Design review of the part built by this model. Coordinates are the model's own, in mm. Coordinates: 2 decimals unless noted, no trailing zeros. Loops run counter-clockwise (first coordinate to the right, second up) from the corner with the lowest first, then second, coordinate; pieces in that order, holes last. Notation, with made-up numbers: (23.5, 88) - (52.5, 88) arc R19 ccw to (52.5, 104) - close; hole circle Ø10 at (19.25, -9). An arc over 180 degrees is marked (long way). Use one line per item in the form item = value. Start each with the question number.
(1) Add section C-C (z = -7). Count the separate pieces of the cut face and the enclosed holes in it, plus the area to 4 significant figures.
(2) Add section B-B (x = 36.25). State the section outline as (y, z) points, plus the area to 3 significant figures.
(3) For L1, parallel to Z at x = 36.25, y = 0.65; L2, parallel to Z at x = 42, y = 0.65; L3, parallel to Z at x = 24.5, y = 1.85, list the stretches that pass through material, from the lowest coordinate up.
(4) Add section A-A (x = 16.9). State the section outline as (y, z) points, plus the area to 3 significant figures.
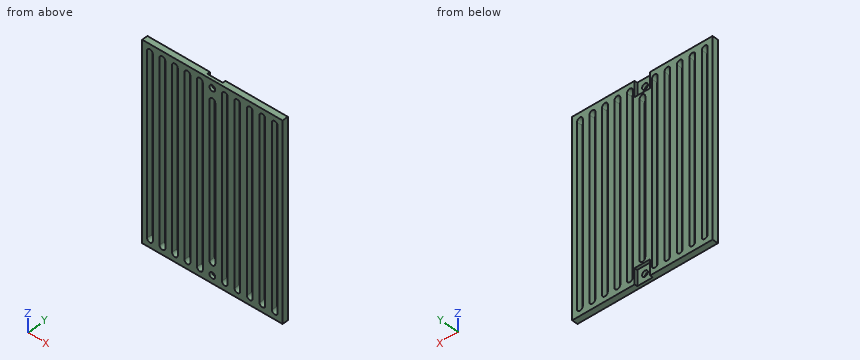
Autodesk Inventor part; units mm, degrees
ref_plane "YZ Plane" through (0, 0, 0) normal (1, 0, 0) x (0, 1, 0)
ref_plane "XZ Plane" through (0, 0, 0) normal (0, 1, 0) x (-1, 0, 0)
ref_plane "XY Plane" through (0, 0, 0) normal (0, 0, 1) x (1, 0, 0)
sketch "Sketch1" plane through (0, 0, 0) normal (0, 1, 0) x (-1, 0, 0)
  line L0 (0, 0) -> (-72.5, 0)
  line L1 (-72.5, 0) -> (-72.5, -100)
  line L2 (-72.5, -100) -> (0, -100)
  line L3 (0, -100) -> (0, 0)
  dimension "d0" = 72.5
  dimension "d1" = 100
extrude "Extrusion1" add sketch "Sketch1" along normal blind 3
sketch "Sketch11" plane through (0, 3, 0) normal (0, 1, 0) x (1, 0, 0)
  point P0 (0, 0)
sketch "Sketch13" plane through (0, 3, 0) normal (0, 1, 0) x (1, 0, 0)
  line L0 (0, 0) -> (72.5, 0)
  line L1 (36.25, 0) -> (36.25, 8)
  line L2 (36.25, 8) -> (32.25, 8)
  line L3 (32.25, 8) -> (32.25, 0)
  line L4 (36.25, 0) -> (32.25, 0)
  line L5 (36.25, 0) -> (40.25, 0)
  line L6 (40.25, 0) -> (40.25, 8)
  line L7 (40.25, 8) -> (36.25, 8)
  line L8 (72.5, 100) -> (0, 100)
  line L9 (36.25, 100) -> (32.25, 100)
  line L10 (32.25, 100) -> (32.25, 92)
  line L11 (32.25, 92) -> (40.25, 92)
  line L12 (40.25, 92) -> (40.25, 100)
  line L13 (40.25, 100) -> (36.25, 100)
  line L14 (72.5, 0) -> (72.5, 100)
  dimension "d190" = 8
  dimension "d191" = 4
  dimension "d192" = 4
  dimension "d193" = 8
extrude "Extrusion11" cut sketch "Sketch13" against normal blind 1.5
sketch "Sketch14" plane through (0, 1.5, 0) normal (0, 1, 0) x (1, 0, 0)
  line L0 (0, 0) -> (72.5, 0)
  line L1 (40.25, 8) -> (32.25, 8)
  line L2 (32.25, 8) -> (32.25, 0)
  line L3 (32.25, 0) -> (40.25, 0)
  line L4 (40.25, 0) -> (40.25, 8)
  line L5 (72.5, 100) -> (0, 100)
  line L6 (40.25, 100) -> (32.25, 100)
  line L7 (32.25, 100) -> (32.25, 92)
  line L8 (32.25, 92) -> (40.25, 92)
  line L9 (40.25, 92) -> (40.25, 100)
  line L10 (72.5, 46) -> (64.5, 46)
  line L11 (64.5, 46) -> (64.5, 54)
  line L12 (72.5, 46) -> (64.5, 46)
  line L13 (64.5, 46) -> (64.5, 54)
  line L14 (64.5, 54) -> (72.5, 54)
  line L15 (72.5, 54) -> (72.5, 46)
  circle A0 centre (36.25, 4) radius 1.5
  circle A1 centre (36.25, 96) radius 1.5
  circle A2 centre (68.5, 50) radius 1.5
  dimension "d199" = 8
  dimension "d200" = 8
  dimension "d201" = 3
  dimension "d202" = 3
  dimension "d203" = 3
extrude "Extrusion12" cut sketch "Sketch14" against normal blind 1.5 contours A0 | A1 | A2
sketch "Sketch15" plane through (0, 3, 0) normal (0, 1, 0) x (1, 0, 0)
  circle A0 centre (36.25, 4) radius 1.5
  line L0 (0, 100) -> (0, 0)
  circle A1 centre (36.25, 96) radius 1.5
  line L1 (32.25, 8) -> (40.25, 8)
  arc A2 (2.5, 4) -> (5.5, 4) centre (4, 4) ccw
  arc A3 (15.4, 4) -> (18.4, 4) centre (16.9, 4) ccw
  arc A4 (21.85, 4) -> (24.85, 4) centre (23.35, 4) ccw
  arc A5 (28.3, 4) -> (31.3, 4) centre (29.8, 4) ccw
  arc A6 (41.2, 4) -> (44.2, 4) centre (42.7, 4) ccw
  arc A7 (47.65, 4) -> (50.65, 4) centre (49.15, 4) ccw
  arc A8 (54.1, 4) -> (57.1, 4) centre (55.6, 4) ccw
  arc A9 (60.55, 4) -> (63.55, 4) centre (62.05, 4) ccw
  arc A10 (67, 4) -> (70, 4) centre (68.5, 4) ccw
  arc A11 (70, 96) -> (67, 96) centre (68.5, 96) ccw
  arc A12 (63.55, 96) -> (60.55, 96) centre (62.05, 96) ccw
  arc A13 (57.1, 96) -> (54.1, 96) centre (55.6, 96) ccw
  arc A14 (50.65, 96) -> (47.65, 96) centre (49.15, 96) ccw
  arc A15 (44.2, 96) -> (41.2, 96) centre (42.7, 96) ccw
  arc A16 (31.3, 96) -> (28.3, 96) centre (29.8, 96) ccw
  arc A17 (24.85, 96) -> (21.85, 96) centre (23.35, 96) ccw
  arc A18 (18.4, 96) -> (15.4, 96) centre (16.9, 96) ccw
  arc A19 (5.5, 96) -> (2.5, 96) centre (4, 96) ccw
  line L2 (8.95, 16.45) -> (8.95, 83.55)
  line L3 (11.95, 83.55) -> (11.95, 16.45)
  line L4 (15.4, 4) -> (15.4, 96)
  line L5 (18.4, 96) -> (18.4, 4)
  line L6 (21.85, 96) -> (21.85, 4)
  line L7 (24.85, 4) -> (24.85, 96)
  line L8 (28.3, 96) -> (28.3, 4)
  line L9 (31.3, 4) -> (31.3, 96)
  line L10 (41.2, 96) -> (41.2, 4)
  line L11 (44.2, 4) -> (44.2, 96)
  line L12 (47.65, 96) -> (47.65, 4)
  line L13 (50.65, 4) -> (50.65, 96)
  line L14 (54.1, 96) -> (54.1, 4)
  line L15 (57.1, 4) -> (57.1, 96)
  line L16 (60.55, 96) -> (60.55, 4)
  line L17 (63.55, 4) -> (63.55, 96)
  line L18 (67, 43.55) -> (67, 4)
  line L19 (70, 4) -> (70, 43.55)
  line L20 (67, 56.45) -> (67, 96)
  line L21 (70, 96) -> (70, 56.45)
  line L22 (36.25, 4) -> (36.25, 10.45)
  arc A20 (34.75, 10.45) -> (37.75, 10.45) centre (36.25, 10.45) ccw
  line L23 (36.25, 96) -> (36.25, 89.55)
  arc A21 (37.75, 89.55) -> (34.75, 89.55) centre (36.25, 89.55) ccw
  line L24 (34.75, 10.45) -> (34.75, 89.55)
  line L25 (37.75, 89.55) -> (37.75, 10.45)
  arc A22 (8.95, 4) -> (11.95, 4) centre (10.45, 4) ccw
  arc A23 (11.95, 96) -> (8.95, 96) centre (10.45, 96) ccw
  line L26 (8.95, 96) -> (8.95, 83.55)
  line L27 (11.95, 96) -> (11.95, 83.55)
  line L28 (8.95, 16.45) -> (8.95, 4)
  line L29 (11.95, 16.45) -> (11.95, 4)
  line L30 (5.5, 4) -> (5.5, 43.55)
  line L31 (5.5, 56.45) -> (5.5, 96)
  line L32 (2.5, 96) -> (2.5, 56.45)
  line L33 (2.5, 43.55) -> (2.5, 4)
  line L34 (2.5, 56.45) -> (2.5, 43.55)
  line L35 (5.5, 43.55) -> (5.5, 56.45)
  line L36 (67, 56.45) -> (67, 43.55)
  line L37 (70, 43.55) -> (70, 56.45)
  dimension "d216" = 3
  dimension "d217" = 3
  dimension "d218" = 3
  dimension "d219" = 3
  dimension "d220" = 3
  dimension "d221" = 3
  dimension "d225" = 3
  dimension "d226" = 3
  dimension "d227" = 3
  dimension "d228" = 3
  dimension "d229" = 3
  dimension "d230" = 3
  dimension "d231" = 3
  dimension "d232" = 3
  dimension "d233" = 3
  dimension "d242" = 6.45
  dimension "d243" = 3
  dimension "d244" = 6.45
  dimension "d245" = 3
  dimension "d248" = 3
  dimension "d249" = 3
extrude "Extrusion13" cut sketch "Sketch15" against normal blind 3 contours A20 L24 A21 L25 | L33 L34 L32 A19 L31 L35 L30 A2 | L4 A18 L5 A3 | L6 A17 L7 A4 | L8 A16 L9 A5 | L10 A15 L11 A6 | L12 A14 L13 A7 | L14 A13 L15 A8 | L16 A12 L17 A9 | L18 L36 L20 A11 L21 L37 L19 A10 | L2 L26 A23 L27 L3 L29 A22 L28
sketch "Sketch16" plane through (0, 3, 0) normal (0, 1, 0) x (1, 0, 0)
  point P0 (0, 0)
properties part number "Tray middle"
Computed values:
q1.separate_pieces = 11
q1.enclosed_holes = 0
q1.area = 115.5 mm^2
q2.outline = (0, -100) - (1.5, -100) - (1.5, -97.5) - (0, -97.5) - close; (0, -94.5) - (1.5, -94.5) - (1.5, -92) - (3, -92) - (3, -91.05) - (0, -91.05) - close; (0, -8.95) - (3, -8.95) - (3, -8) - (1.5, -8) - (1.5, -5.5) - (0, -5.5) - close; (0, -2.5) - (1.5, -2.5) - (1.5, 0) - (0, 0) - close
q2.area = 20.7 mm^2
q3.L1 = -100 to -97.5, -94.5 to -91.05, -8.95 to -5.5, -2.5 to 0
q3.L2 = -100 to -97.33, -2.67 to 0
q3.L3 = -100 to -96.96, -3.04 to 0
q4.outline = (0, -100) - (3, -100) - (3, -97.5) - (0, -97.5) - close; (0, -2.5) - (3, -2.5) - (3, 0) - (0, 0) - close
q4.area = 15.0 mm^2
